Build history of the part. All positions in model axes, mm. Face numbers are marked on the shaded views. Give positions to 0.01 mm unless a question says otherwise; leave off trailing zeros. Loops run counter-clockwise (first coordinate to the right, second up) from the corner with the lowest first, then second, coordinate; pieces in that order, holes last. Notation, with made-up numbers: M 11,39.5 L 39,39.5 A28 ccw 39,66.5 Z; hole C -12.5,53.25 d3. An arc over 180 degrees is marked long. Answer in a Markdown table with one row per item. Add a question column.
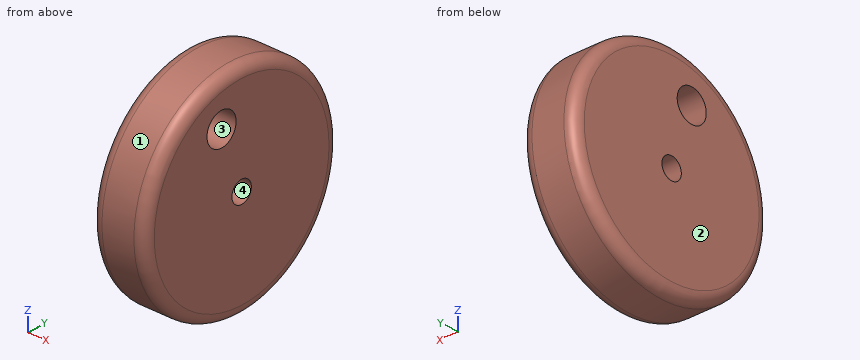
```python
from build123d import *

# Parameters (mm, degrees)
F0_R     = 50
F0_R_2   = 7.496671
F0_R_3   = 5
F1_DEPTH = 25
F2_R     = 5


with BuildPart() as f1:
    # F0 (on Right) → F1 (new body)
    with BuildSketch(Plane.YZ):
        Circle(F0_R)
        with Locations((-10.344213, 29.099595)):
            Circle(F0_R_2, mode=Mode.SUBTRACT)
        Circle(F0_R_3, mode=Mode.SUBTRACT)
    extrude(amount=F1_DEPTH)

    # F2
    f2_edges = [f1.edges().sort_by_distance(p)[0] for p in [
        (25, -50, 0),
        (0, -50, 0),
    ]]
    fillet(f2_edges, radius=F2_R)


solid = f1.part
```
(1) Pin check, flat tips, straight feed: pin 1 (10 mm diameter, centred on x = 4, y = 38.5, fed in from -Z); pin 2 (2 mm diameter, centred on x = 14.5, z = 39.5, fed in from -Y); pin 3 (17 mm diameter, centred on y = -10.34, z = 29.1, fed in from -X); pin 4 (1.5 mm diameter, centred on x = 12.5, z = -24.5, fed in from -Y). Stop position of each tip, or through.
(2) Pull direction Y, two halves, no side cores. Call the marked faces 1, 2, 3 and 4: +Y half, -Y half, draft (parallel to the pull), parting line (faces both ways), or undercut.
(3) Wall check: line 1 (Z direction, x = 1.5, y = -6); line 2 (X direction, y = 17, z = 42); line 3 (Z direction, x = 10.25, y = -2.5). Give the ranges that are in metal, low to high.
(4) Slice it at A-A, the plane z = 0. Give the cut face in (x, y), then the cut area to 3 significant figures.
(5) Slice it at C-C, the plane x = 3.75. Give the cut face in (y, z), then the cut area to 3 significant figures.
Solution:
| question | item | result |
|---|---|---|
| 1 | pin 1 | z = -37.06 |
| 1 | pin 2 | y = -31.9 |
| 1 | pin 3 | x = 0 |
| 1 | pin 4 | y = -44 |
| 2 | face 1 | parting line |
| 2 | face 2 | draft |
| 2 | face 3 | undercut |
| 2 | face 4 | undercut |
| 3 | line 1 | -48.2 to 22.99, 35.21 to 48.2 |
| 3 | line 2 | 0.01 to 24.99 |
| 3 | line 3 | -49.94 to -4.33, 4.33 to 49.94 |
| 4 | outline | M 0,-45 A5 ccw 5,-50 L 20,-50 A5 ccw 25,-45 L 25,-5 L 0,-5 Z; M 0,5 L 25,5 L 25,45 A5 ccw 20,50 L 5,50 A5 ccw 0,45 Z |
| 4 | area | 2,230 mm^2 |
| 5 | outline | C 0,0 d99.68; hole C -10.34,29.1 d14.99; hole C 0,0 d10 |
| 5 | area | 7,550 mm^2 |
